```python
from build123d import *

# Parameters (mm, degrees)
EXTRUDE_1_DEPTH = 12.5
FILLET_1_R      = 6


with BuildPart() as part:
    # 草图1 → 凸台-拉伸1 (new, symmetric)
    with BuildSketch(Plane.XY):
        with BuildLine():
            Line((0, 0), (26, 0))
            ThreePointArc((26, 0), (27.468456661, -6.472815065), (31.586311315, -11.678290343))
            ThreePointArc((31.586311315, -11.678290343), (67.528745318, -55.48682347), (83, -110))
            Line((83, -110), (25, -110))
            ThreePointArc((25, -110), (15.68286649, -69.005354222), (0, -30))
            Line((0, -30), (0, 0))
        make_face()
    extrude(amount=EXTRUDE_1_DEPTH, both=True)

    # 圆角1
    fillet_1_edges = [part.edges().sort_by_distance(p)[0] for p in [
        (83, -110, 0),
        (25, -110, 0),
        (54, -110, 12.5),
        (67.528745318, -55.48682347, 12.5),
        (27.468456661, -6.472815065, 12.5),
        (27.468456661, -6.472815065, -12.5),
        (67.528745318, -55.48682347, -12.5),
        (54, -110, -12.5),
        (15.68286649, -69.005354222, -12.5),
        (15.68286649, -69.005354222, 12.5),
    ]]
    fillet(fillet_1_edges, radius=FILLET_1_R)


solid = part.part
```
Source: CAD feature listing. Evaluate the final solid. Frame: model axes, mm. Coordinates: 2 decimals unless noted, no trailing zeros. Write each loop counter-clockwise with the first axis right and the second up, starting at its lowest first coordinate (ties: lowest second). Pieces come first, ordered by that corner, then holes. Notation, with made-up numbers: (54, 87.25) - (108, 87.25) arc R25 cw to (108, 125.25) - close; hole circle Ø10 at (31.25, 8.25). An arc over 180 degrees is marked (long way). Answer as a JSON object with one key per item and string values.
Q1. Section query A-A, the plane z = -2. Output: boundary loops of the cut face in (x, y).
Ans:
{"outline": "(0, -30) arc R265 cw to (24.22, -104.98) arc R6 ccw to (30.14, -110) - (76.4, -110) arc R6 ccw to (82.36, -103.28) arc R139 ccw to (31.59, -11.68) arc R15 cw to (26, 0) - (0, 0) - close"}
Q2. First-contact query: pin 1 Ø3 at (x, z) = (66, -8.5) entering from +Y; pin 2 Ø3 at (y, z) = (-92.5, 6.5) entering from -X; pin 3 Ø6 at (y, z) = (-55, 9.5) entering from +X. Flat tips, straight axial feed; report the tip coordinate or a pass-through.
Ans:
{"pin 1": "stops at y = -50.53", "pin 2": "stops at x = 21.53", "pin 3": "stops at x = 68.4"}
Q3. Material intervals for line 1 (X direction, y = -46, z = -10.75); line 2 (Y direction, x = 40, z = 6.25); line 3 (X direction, y = -14, z = 11.5), sorted ascending. Write a range as [from, to].
Ans:
{"line 1": "x = [9.22, 59.99]", "line 2": "y = [-110, -19.04]", "line 3": "x = [0, 30.19]"}
Q4. Section query B-B, the plane z = -9.5. Output: boundary loops of the cut face in (x, y).
Ans:
{"outline": "(0, -28.21) arc R265.8 cw to (25.01, -104.84) arc R5.2 ccw to (30.14, -109.2) - (76.4, -109.2) arc R5.2 ccw to (81.56, -103.38) arc R138.2 ccw to (31.08, -12.3) arc R15.8 cw to (25.2, 0) - (0, 0) - close"}
